from build123d import *

# Parameters (mm, degrees)
SKETCH1_W                   = 69.85
SKETCH1_H                   = 101.6
BASE_FLANGE1_DEPTH          = 3.175
EDGE_FLANGE1_DEPTH          = 69.85
F_5_0_2055_DIAMETER_HOLE1_D = 5.2197


# Sheet-metal steps are written as plain solids
with BuildPart() as part:
    # Sketch1 → Base-Flange1 (new body)
    with BuildSketch(Plane(origin=(0, 0, 0), x_dir=(1, 0, 0), z_dir=(0, 1, 0))):
        with Locations((34.925, 50.8)):
            Rectangle(SKETCH1_W, SKETCH1_H)
    extrude(amount=-BASE_FLANGE1_DEPTH)

    # Edge-Flange1 section (across the edge) → Edge-Flange1 (add)
    with BuildSketch(Plane(origin=(0, 0, 3.9116), x_dir=(0, 0, -1), z_dir=(1, 0, 0))):
        with BuildLine():
            Line((-3.175, 0.7366), (-3.175, 22.225))
            Line((-3.175, 22.225), (0, 22.225))
            Line((0, 22.225), (0, 0.7366))
            ThreePointArc((0, 0.7366), (0.215745145, 0.215745145), (0.7366, 0))
            Line((0.7366, 0), (3.9116, 0))
            Line((3.9116, 0), (3.9116, -3.175))
            Line((3.9116, -3.175), (0.7366, -3.175))
            ThreePointArc((0.7366, -3.175), (-2.029318885, -2.029318885), (-3.175, 0.7366))
        make_face()
    extrude(amount=EDGE_FLANGE1_DEPTH)

    # #5 (0.2055) Diameter Hole1 (through all)
    with Locations(Plane.XZ.offset(3.175)):
        with Locations((33.3375, -34.1884), (23.8125, -62.7634), (33.3375, -72.2884), (57.15, -84.9884), (57.15, -40.5384), (9.525, -40.5384), (9.525, -84.9884)):
            Hole(F_5_0_2055_DIAMETER_HOLE1_D / 2)


solid = part.part
Design review of the part built by this model. Coordinates are the model's own, in mm. A direction names the side the tool comes from. Coordinates: 2 decimals unless noted, no trailing zeros. Order: outer loops, then holes, each group sorted by start corner. A loop starts at its lowest first (then second) coordinate and runs counter-clockwise, first axis right, second up. Notation, with made-up numbers: (29.25, -12) -> (41.25, -12) arc R13 ccw to (41.25, 3) -> close; hole circle Ø1 at (24, -1.5). An arc over 180 degrees is marked (long way). Use one line per item in the form item = value. Start each with the question number.
(1) Add section C-C on x = 49. State the section outline as (y, z) points (3 decimals).
(2) Add section B-B on y = -1.25. Give the number of separate pieces and of enclosed holes in the cut face, plus the area to 3 significant figures.
(3) Add section A-A on x = 57.15. State the section outline as (y, z) points (3 decimals), plus the area to 3 significant figures.
(4) For probe 1 along Z at (x, y) = (57.15, -1.6); probe 2 along Y at (x, z) = (28, -10.5) (3 decimals); probe 3 along Z at (x, y) = (57, 12), list the stretches that pass through material, from the lowest coordinate up.
(5) For faces 1 (the cylindrical face through (21.4, -1.57, -63.76)), 2 (the flat face through (34, 0, -48)), list the 3-axis set-ups (+Z, -Z, +X, -X, +Y, -Y) from which the entire face can be reached by the end or side of a thin tool; tool diameter is ignored.
(6) Insertion check: pin 1 (3 mm diameter, centred on x = 59.5, y = 16, fed in from -Z); pin 2 (6 mm diameter, centred on x = 33.34, z = -34.19, fed in from -Y) (3 decimals). Each pin has a flat end and moves straight along its axis. Give the tip position at first contact, or say it passes through.
(7) Add section D-D on z = -29.5. State the section outline as (x, y) points (3 decimals), plus the area to 3 significant figures.
(8) The part is to be moulded in two halves that separate along Z. For faces 3 (the cylindrical face through (33.903, -1.565, -74.836)), 4 (the flat face through (34, 11, 7.087)), 5 (the flat face through (34, -2, -101.6)), say which applies: +Z half, -Z half, draft (parallel to the pull), parting line (faces both ways), or undercut.
Answer block:
q1.outline = (-3.175, -101.6) -> (0, -101.6) -> (0, 3.175) arc R0.737 cw to (0.737, 3.912) -> (22.225, 3.912) -> (22.225, 7.087) -> (0.737, 7.087) arc R3.912 ccw to (-3.175, 3.175) -> close
q2.separate_pieces = 1
q2.enclosed_holes = 7
q2.area = 7,400 mm²
q3.outline = (-3.175, -101.6) -> (0, -101.6) -> (0, -87.598) -> (-3.175, -87.598) -> close; (-3.175, -82.379) -> (0, -82.379) -> (0, -43.148) -> (-3.175, -43.148) -> close; (-3.175, -37.929) -> (0, -37.929) -> (0, 3.175) arc R0.737 cw to (0.737, 3.912) -> (22.225, 3.912) -> (22.225, 7.087) -> (0.737, 7.087) arc R3.912 ccw to (-3.175, 3.175) -> close
q3.area = 379 mm²
q4.probe_1 = -101.6 to -87.6, -82.38 to -43.15, -37.93 to 6.31
q4.probe_2 = -3.175 to 0
q4.probe_3 = 3.91 to 7.09
q5.face_1 = +Y, -Y
q5.face_2 = -Z, +X, -X, +Y
q6.pin_1 = 3.91
q6.pin_2 = -3.175
q7.outline = (0, -3.175) -> (69.85, -3.175) -> (69.85, 0) -> (0, 0) -> close
q7.area = 222 mm²
q8.face_3 = undercut
q8.face_4 = +Z half
q8.face_5 = -Z half
